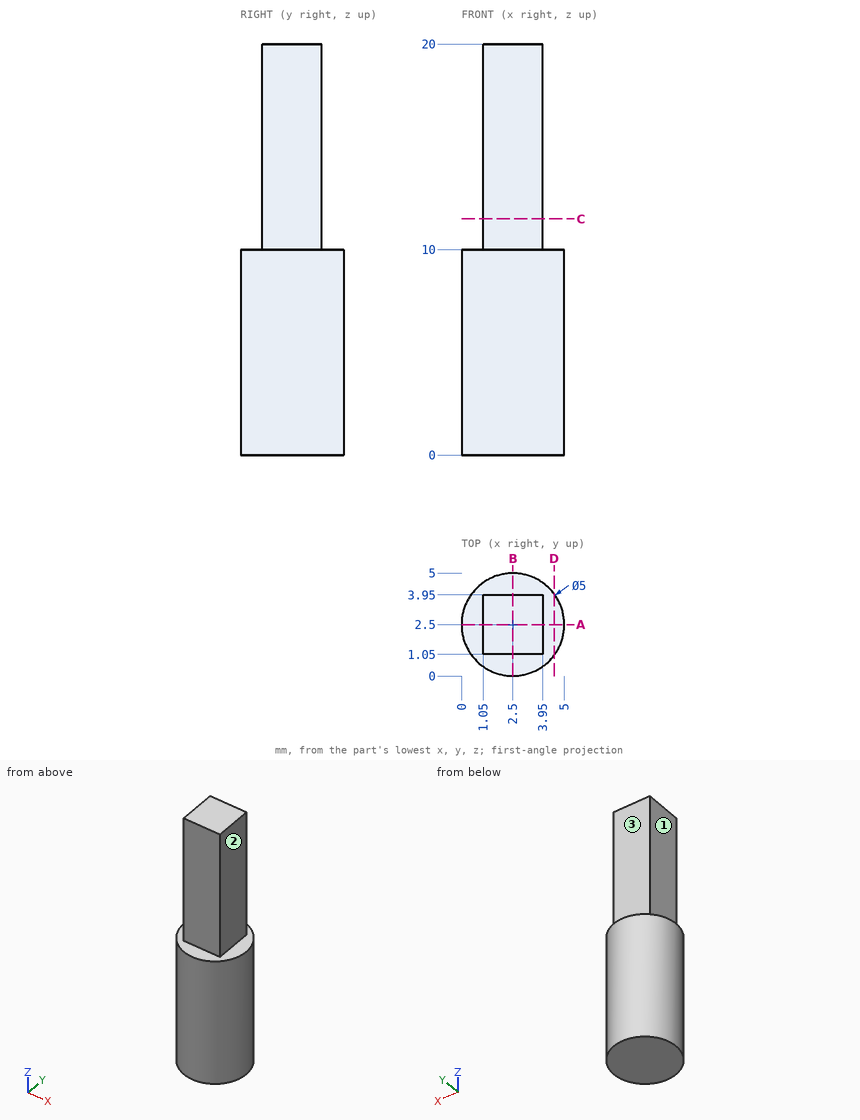
Part print with two shaded views. Sizes in mm from the minimum x, y, z corner. A direction names the side the tool comes from. Round coordinates to 2 decimals unless told otherwise and drop trailing zeros. Write each loop counter-clockwise with the first axis right and the second up, starting at its lowest first coordinate (ties: lowest second). Pieces come first, ordered by that corner, then holes. Notation, with made-up numbers: M 53.25,56.25 L 76.25,56.25 A26 cw 76.25,87.25 Z; hole C 21,-29.75 d1. An arc over 180 degrees is marked long. Use CSV: the item, a comma, the result in double quotes.
1. Flat gauge pins, fed straight in: pin 1 (1.5 mm diameter, centred on y = 3, z = 12.5, fed in from -X); pin 2 (1.5 mm diameter, centred on x = 3, z = 16.5, fed in from +Y); pin 3 (1 mm diameter, centred on y = 4, z = 7, fed in from +X). Where does each tip first touch, or does it go through?
Reply:
pin 1,"stops at x = 1.05"
pin 2,"stops at y = 3.95"
pin 3,"stops at x = 4.79"
2. Wall check: probe 1 along Z at (x, y) = (0.55, 2.3); probe 2 along X at (y, z) = (2.65, 3.5); probe 3 along X at (y, z) = (3.8, 12). Give the ranges that are in metal, low to high. Write a range as from..to.
Reply:
probe 1,"z = 0..10"
probe 2,"x = 0..5"
probe 3,"x = 1.05..3.95"
3. Saw through at C-C (z = 11.5). Give the cut face in (x, y).
Reply:
outline,"M 1.05,1.05 L 3.95,1.05 L 3.95,3.95 L 1.05,3.95 Z"
4. Saw through at D-D (x = 4.5). Give the cut face in (y, z).
Reply:
outline,"M 1,0 L 4,0 L 4,10 L 1,10 Z"
5. Saw through at A-A (y = 2.5). Give the cut face in (x, z).
Reply:
outline,"M 0,0 L 5,0 L 5,10 L 3.95,10 L 3.95,20 L 1.05,20 L 1.05,10 L 0,10 Z"
6. Tool access for the marked faces 1, 2 and 3: list every direction of +Z, -Z, +X, -X, +Y, -Y with a clear straight run to the whole face (end or side of a thin tool).
Reply:
face 1,"+Z, -X, +Y, -Y"
face 2,"+Z, +X, +Y, -Y"
face 3,"+Z, +X, -X, +Y"
